Source: three-view drawing plus pictorial views. Frame: mm from the lowest corner of the part. A direction names the side the tool comes from. Give positions to 0.01 mm unless a question says otherwise; leave off trailing zeros. Loops run counter-clockwise (first coordinate to the right, second up) from the corner with the lowest first, then second, coordinate; pieces in that order, holes last. Notation, with made-up numbers: (32.5, 56) - (56.5, 56) arc R25 ccw to (56.5, 95) - close; hole circle Ø8 at (23.5, 12). An arc over 180 degrees is marked (long way). One line per item, written item: value.
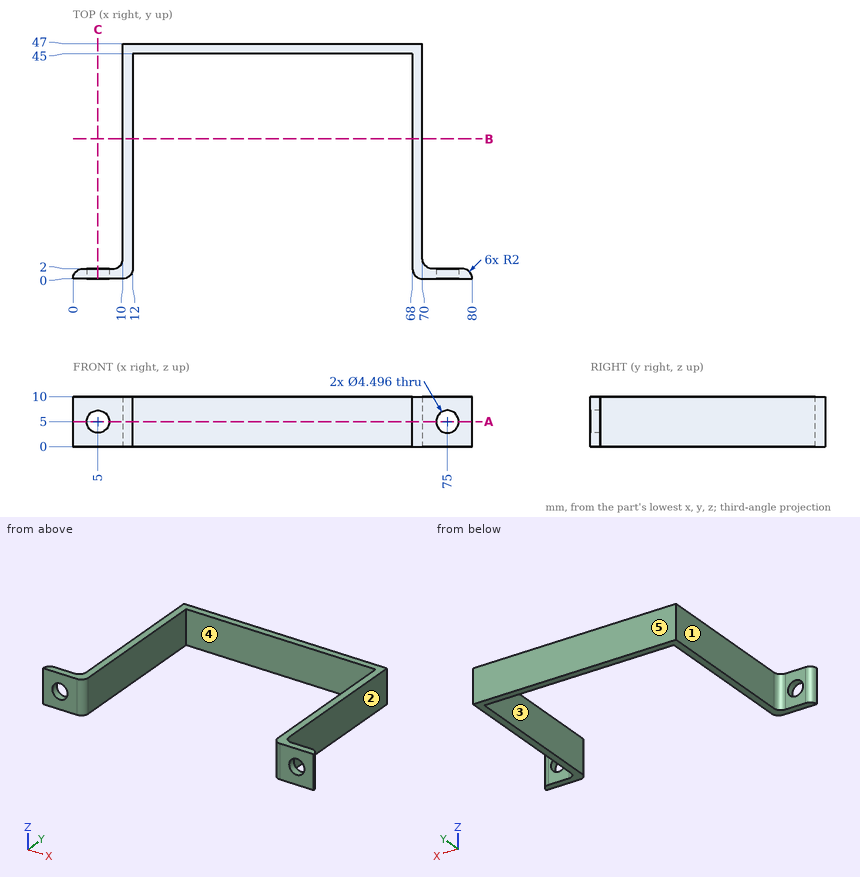
Item 1: Section C-C, the plane x = 5. Output: boundary loops of the cut face in (y, z).
Verdict:
outline: (0, 0) - (2, 0) - (2, 2.75) - (0, 2.75) - close; (0, 7.25) - (2, 7.25) - (2, 10) - (0, 10) - close
Item 2: Material intervals for L1, parallel to Z at x = 5, y = 0.7; L2, parallel to X at y = 24.5, z = 1.75; L3, parallel to Y at x = 15.5, z = 4, sorted ascending.
Verdict:
L1: z = 0 to 2.75, 7.25 to 10
L2: x = 10 to 12, 68 to 70
L3: y = 45 to 47
Item 3: Access query for the marked faces 4 and 5. Directions: +Z, -Z, +X, -X, +Y, -Y. A direction counts if a zero-diameter tool reaches every point of the face in a straight line with its end or side. Return the directions, or none.
Verdict:
face 4: +Z, -Z, -Y
face 5: +Z, -Z, +X, -X, +Y
Item 4: Pin query (flat end, axial travel): P1, Ø3, axis at y = 28.5, z = 3, coming from the -X side; P2, Ø1.5, axis at y = 12, z = 8, coming from the +X side; P3, Ø1.5, axis at x = 44, z = 1, coming from the -Y side. Return the tip coordinate at first contact, or that it passes through.
Verdict:
P1: stops at x = 10
P2: stops at x = 70
P3: stops at y = 45
Item 5: Section B-B, the plane y = 28. Output: boundary loops of the cut face in (x, z), and give its area (3 significant figures).
Verdict:
outline: (10, 0) - (12, 0) - (12, 10) - (10, 10) - close; (68, 0) - (70, 0) - (70, 10) - (68, 10) - close
area: 40.0 mm^2
Item 6: Draft query along X for the marked faces 1, 2 and 3. Return one class per face: pulls with the +X half, pulls with the -X half, needs draft (parallel to the pull), parting line crosses it, or undercut.
Verdict:
face 1: pulls with the -X half
face 2: pulls with the +X half
face 3: undercut
Item 7: Section A-A, the plane z = 5. Count the separate pieces of the cut face and the enclosed holes in it, and give its area (3 significant figures).
Verdict:
separate pieces: 3
enclosed holes: 0
area: 320 mm^2
